from build123d import *

# Parameters (mm, degrees)
F0_R      = 14
F1_DEPTH  = 32
F2_R      = 4.5
F3_DEPTH  = 2
F4_R      = 2
F5_DEPTH  = 13
F6_SIZE   = 0.5
F7_R      = 2
F8_DEPTH  = 5
F10_R     = 4
F11_DEPTH = 6


with BuildPart() as f1:
    # F0 (on Top) → F1 (new body)
    with BuildSketch(Plane.XY):
        Circle(F0_R)
    extrude(amount=F1_DEPTH)

    # F2 (on face) → F3 (join)
    with BuildSketch(Plane.XY.offset(32)):
        Circle(F2_R)
    extrude(amount=F3_DEPTH)

    # F4 (on face) → F5 (join)
    with BuildSketch(Plane.XY.offset(34)):
        Circle(F4_R)
    extrude(amount=F5_DEPTH)

    # F6
    f6_edges = [f1.edges().sort_by_distance(p)[0] for p in [
        (-2, 0, 47),
    ]]
    chamfer(f6_edges, length=F6_SIZE)

    # F7 (on face) → F8 (cut)
    with BuildSketch(Plane(origin=(0, 0, 0), x_dir=(1, 0, 0), z_dir=(0, 0, -1))):
        with Locations((-8, 0)):
            Circle(F7_R)
        with Locations((8, 0)):
            Circle(F7_R)
        with Locations((0, 9.5)):
            Circle(F7_R)
        with Locations((0, -9.5)):
            Circle(F7_R)
    extrude(amount=-F8_DEPTH, mode=Mode.SUBTRACT)

    # F10 (on face) → F11 (join)
    with BuildSketch(Plane.XY.offset(34)):
        Circle(F10_R)
    extrude(amount=F11_DEPTH)


solid = f1.part
Design review of the part built by this model. Coordinates are the model's own, in mm. A direction names the side the tool comes from. Coordinates: 2 decimals unless noted, no trailing zeros. Loops run counter-clockwise (first coordinate to the right, second up) from the corner with the lowest first, then second, coordinate; pieces in that order, holes last.
Item 1: Wall thickness on L1, parallel to Y at x = 8, z = 3.5; L2, parallel to Z at x = 4.75, y = 3; L3, parallel to X at y = -9.5, z = 1.6: over which ranges is each line inside the solid? List them lowest first.
Completed:
L1: y = -11.49 to -2, 2 to 11.49
L2: z = 0 to 32
L3: x = -10.28 to -2, 2 to 10.28
Item 2: Add section B-B (y = 0). Write out the cut boundary in (x, z).
Completed:
outline: (-14, 0) - (-10, 0) - (-10, 5) - (-6, 5) - (-6, 0) - (6, 0) - (6, 5) - (10, 5) - (10, 0) - (14, 0) - (14, 32) - (4.5, 32) - (4.5, 34) - (4, 34) - (4, 40) - (2, 40) - (2, 46.5) - (1.5, 47) - (-1.5, 47) - (-2, 46.5) - (-2, 40) - (-4, 40) - (-4, 34) - (-4.5, 34) - (-4.5, 32) - (-14, 32) - close
Item 3: Add section D-D (x = -8). Write out the cut boundary in (y, z).
Completed:
outline: (-11.49, 0) - (-2, 0) - (-2, 5) - (2, 5) - (2, 0) - (11.49, 0) - (11.49, 32) - (-11.49, 32) - close
Item 4: Draft analysis for pull direction X (two halves, no side actions). For faces 1 (the cylindrical face through (-0.59, 4.46, 32.99)), 2 (the flat face through (0, 0, 47)), 3 (the cylindrical face through (-0.26, -11.483, 2.465)), state which applies: pulls with the +X half, pulls with the -X half, needs draft (parallel to the pull), parting line crosses it, or undercut.
Completed:
face 1: parting line crosses it
face 2: needs draft
face 3: undercut
Item 5: For faces 4 (the flat face through (-3.3, 3.3, 32)), 5 (the flat face through (0, 0, 0)), 6 (the flat face through (0, 9, 5)), list the 3-axis set-ups (+Z, -Z, +X, -X, +Y, -Y) from which the entire face can be reached by the end or side of a thin tool; tool diameter is ignored.
Completed:
face 4: +Z
face 5: -Z, +X, -X, +Y, -Y
face 6: -Z
Item 6: Clearance check with flat-ended pins moving along their axes: pin 1 (4 mm diameter, centred on y = 4, z = 35.5, fed in from -X); pin 2 (1 mm diameter, centred on x = -11, z = 11.5, fed in from +Y); pin 3 (6.5 mm diameter, centred on x = 0, y = 9.5, fed in from +Z). State where each tip first meets the part, or that it passes through.
Completed:
pin 1: stops at x = -3.62
pin 2: stops at y = 9.26
pin 3: stops at z = 32
Item 7: Add section C-C (z = 19). Write out the cut boundary in (x, y), and give its area (3 significant figures).
Completed:
outline: circle Ø28 at (0, 0)
area: 616 mm2
Item 8: Add section A-A (x = 0). Write out the cut boundary in (y, z).
Completed:
outline: (-14, 0) - (-11.5, 0) - (-11.5, 5) - (-7.5, 5) - (-7.5, 0) - (7.5, 0) - (7.5, 5) - (11.5, 5) - (11.5, 0) - (14, 0) - (14, 32) - (4.5, 32) - (4.5, 34) - (4, 34) - (4, 40) - (2, 40) - (2, 46.5) - (1.5, 47) - (-1.5, 47) - (-2, 46.5) - (-2, 40) - (-4, 40) - (-4, 34) - (-4.5, 34) - (-4.5, 32) - (-14, 32) - close
